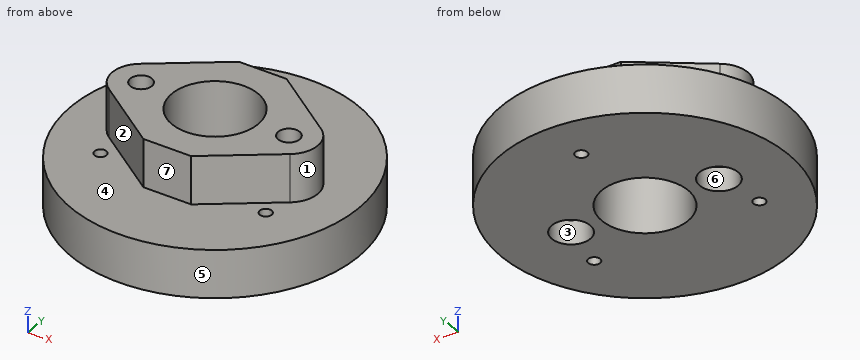
from build123d import *

# Parameters (mm, degrees)
SKETCH_1_R               = 30
SKETCH_1_R_2             = 9
SKETCH_1_R_3             = 1.25
EXTRUDE_1_DEPTH          = 10
SKETCH_3_R               = 9
EXTRUDE_2_DEPTH          = 10
CUT_EXTRUDE_1_DEPTH      = 44.588989435
CUT_EXTRUDE_1_DEPTH_BACK = 44.588989435
SKETCH_2_R               = 2.25
SKETCH_4_R               = 4
CUT_EXTRUDE_2_DEPTH      = 5


with BuildPart() as part:
    # 草图1 → 凸台-拉伸1 (new body)
    with BuildSketch(Plane.XY):
        Circle(SKETCH_1_R)
        Circle(SKETCH_1_R_2, mode=Mode.SUBTRACT)
        with Locations((0, 20)):
            Circle(SKETCH_1_R_3, mode=Mode.SUBTRACT)
        with Locations((17.320508076, -10)):
            Circle(SKETCH_1_R_3, mode=Mode.SUBTRACT)
        with Locations((-17.320508076, -10)):
            Circle(SKETCH_1_R_3, mode=Mode.SUBTRACT)
    extrude(amount=EXTRUDE_1_DEPTH)

    # 草图3 → 凸台-拉伸2 (add)
    with BuildSketch(Plane.XY.offset(10)):
        with BuildLine():
            Line((5, 15), (-5, 15))
            Line((-5, 15), (-19.016468159, 4.861527711))
            ThreePointArc((-19.016468159, 4.861527711), (-21.5, 0), (-19.016468159, -4.861527711))
            Line((-19.016468159, -4.861527711), (-5, -15))
            Line((-5, -15), (5, -15))
            Line((5, -15), (19.016468159, -4.861527711))
            ThreePointArc((19.016468159, -4.861527711), (21.5, 0), (19.016468159, 4.861527711))
            Line((19.016468159, 4.861527711), (5, 15))
        make_face()
        Circle(SKETCH_3_R, mode=Mode.SUBTRACT)
    extrude(amount=EXTRUDE_2_DEPTH)

    # 草图2 → 切除-拉伸1 (cut, two sides: drawn at the far end of the back side and taken through both)
    with BuildSketch(Plane.XY.offset(10).offset(-CUT_EXTRUDE_1_DEPTH_BACK)):
        with Locations((-15.5, 0)):
            Circle(SKETCH_2_R)
        with Locations((15.5, 0)):
            Circle(SKETCH_2_R)
    extrude(amount=CUT_EXTRUDE_1_DEPTH + CUT_EXTRUDE_1_DEPTH_BACK, mode=Mode.SUBTRACT)

    # 草图4 → 切除-拉伸2 (cut)
    with BuildSketch(Plane(origin=(0, 0, 0), x_dir=(-1, 0, 0), z_dir=(0, 0, -1))):
        with Locations((-15.5, 0)):
            Circle(SKETCH_4_R)
        with Locations((15.5, 0)):
            Circle(SKETCH_4_R)
    extrude(amount=-CUT_EXTRUDE_2_DEPTH, mode=Mode.SUBTRACT)


solid = part.part
Can you work these out from the model? Positions are in its coordinate system, mm. Face numbers are marked on the shaded views. A direction names the side the tool comes from. Coordinates: 2 decimals unless noted, no trailing zeros. Write each loop counter-clockwise with the first axis right and the second up, starting at its lowest first coordinate (ties: lowest second). Pieces come first, ordered by that corner, then holes. Notation, with made-up numbers: (34.5, 82.25) -> (59.5, 82.25) arc R38 cw to (59.5, 120.25) -> close; hole circle Ø2 at (84.25, 41.25). An arc over 180 degrees is marked (long way). Write each question's results on one line, items separated by ' | '. Start each with the question number.
Q1. Imagine slicing it at C-C (z = 12). Write out the boundary of the cut face in (x, y), then the cut area to 3 significant figures.
Q2. On a 3-axis mill with a long thin cutter (end or side, diameter ignored), from which of +Z, -Z, +X, -X, +Y, -Y can I reach the whole of each face in a straight line? I mean the marked faces 1, 2, 3 and 4. Say none if no direction works.
Q3. Imagine slicing it at B-B (z = 8). Write out the boundary of the cut face in (x, y), then the cut area to 3 significant figures.
Q4. Imagine slicing it at D-D (y = 0). Write out the boundary of the cut face in (x, z), then the cut area to 3 significant figures.
Q5. I'm going to push flat-ended pins straight in: pin 1 (5 mm diameter, centred on x = -2.5, z = 17, fed in from -Y); pin 2 (12 mm diameter, centred on x = 9.5, z = 12, fed in from -Y); pin 3 (8 mm diameter, centred on x = -0.5, z = 6, fed in from +Y); pin 4 (1.5 mm diameter, centred on x = 0, y = 20, fed in from +Z). Where does each tip first touch, or does it pass through?
Q6. Imagine slicing it at A-A (x = 0). Write out the boundary of the cut face in (y, z).
Q7. If I drill on probe 1 along Y at (x, z) = (0, 9.25); probe 2 along Y at (x, z) = (16.5, 1); probe 3 along Y at (x, z) = (0, 11), over which ranges is the centre line in solid material (lowest first)?
Q8. We'd pull the mould along X, two halves only. Please class the marked faces 5, 6 and 7: +X half, -X half, draft (parallel to the pull), parting line (faces both ways), or undercut.
Taken from the geometry:
1) outline: (-19.02, -4.86) -> (-5, -15) -> (5, -15) -> (19.02, -4.86) arc R6 ccw to (19.02, 4.86) -> (5, 15) -> (-5, 15) -> (-19.02, 4.86) arc R6 ccw to start; hole circle Ø4.5 at (-15.5, 0); hole circle Ø18 at (0, 0); hole circle Ø4.5 at (15.5, 0) | area: 604 mm^2
2) face 1: +Z, +X | face 2: +Z, -X, -Y | face 3: -Z | face 4: +Z
3) outline: circle Ø60 at (0, 0); hole circle Ø2.5 at (-17.32, -10); hole circle Ø4.5 at (-15.5, 0); hole circle Ø18 at (0, 0); hole circle Ø2.5 at (0, 20); hole circle Ø4.5 at (15.5, 0); hole circle Ø2.5 at (17.32, -10) | area: 2,530 mm^2
4) outline: (-30, 0) -> (-19.5, 0) -> (-19.5, 5) -> (-17.75, 5) -> (-17.75, 20) -> (-21.5, 20) -> (-21.5, 10) -> (-30, 10) -> close; (-13.25, 5) -> (-11.5, 5) -> (-11.5, 0) -> (-9, 0) -> (-9, 20) -> (-13.25, 20) -> close; (9, 0) -> (11.5, 0) -> (11.5, 5) -> (13.25, 5) -> (13.25, 20) -> (9, 20) -> close; (17.75, 5) -> (19.5, 5) -> (19.5, 0) -> (30, 0) -> (30, 10) -> (21.5, 10) -> (21.5, 20) -> (17.75, 20) -> close | area: 455 mm^2
5) pin 1: stops at y = -15 | pin 2: stops at y = -29.75 | pin 3: stops at y = 30 | pin 4: passes through
6) outline: (-30, 0) -> (-9, 0) -> (-9, 20) -> (-15, 20) -> (-15, 10) -> (-30, 10) -> close; (9, 0) -> (18.75, 0) -> (18.75, 10) -> (15, 10) -> (15, 20) -> (9, 20) -> close; (21.25, 0) -> (30, 0) -> (30, 10) -> (21.25, 10) -> close
7) probe 1: y = -30 to -9, 9 to 18.75, 21.25 to 30 | probe 2: y = -25.05 to -10.94, -9.06 to -3.87, 3.87 to 25.05 | probe 3: y = -15 to -9, 9 to 15
8) face 5: parting line | face 6: undercut | face 7: draft
